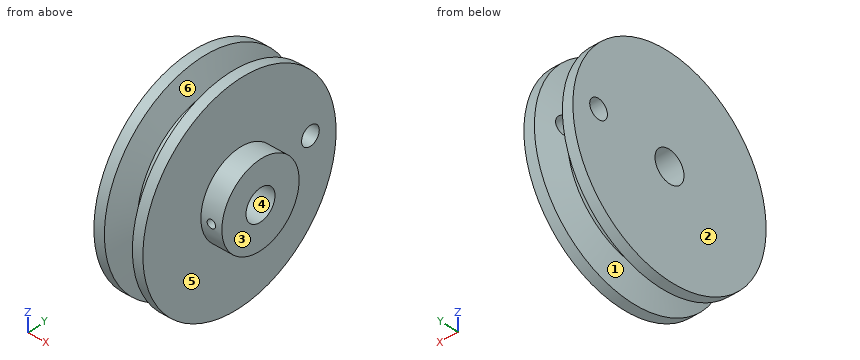
from build123d import *

# Parameters (mm, degrees)
F3_D     = 5.5
F3_DEPTH = 14
F3_TIP   = 1.6523667023
F6_D     = 2.4
F6_DEPTH = 13.4
F6_TIP   = 0.7210327428


with BuildPart() as f1:
    # F0 (on Front) → F1 (revolve)
    with BuildSketch(Plane.XZ):
        Polygon((-7, 30), (-7, 4.5), (13, 4.5), (13, 12), (7, 12), (7, 30), (4, 30), (1.9940651348, 21.9546346889), (-2.0053759773, 22), (-4, 30), align=None)
    revolve(axis=Axis((0, 0, 0), (1, 0, 0)))

    # F3
    with Locations(Plane(origin=(-7, 0, 0), x_dir=(0, -1, 0), z_dir=(-1, 0, 0))):
        with Locations((-22.0234822482, 3.0874926597)):
            Hole(F3_D / 2, depth=F3_DEPTH)
            with Locations((0, 0, -(F3_DEPTH + F3_TIP / 2))):  # 118° drill point
                Cone(0, F3_D / 2, F3_TIP, mode=Mode.SUBTRACT)

    # F6
    with Locations(Plane.XZ.offset(12)):
        with Locations((10, 0)):
            Hole(F6_D / 2, depth=F6_DEPTH)
            with Locations((0, 0, -(F6_DEPTH + F6_TIP / 2))):  # 118° drill point
                Cone(0, F6_D / 2, F6_TIP, mode=Mode.SUBTRACT)


solid = f1.part
Verification items for the finished model (mm, model axes). Face numbers are marked on the shaded views. A direction names the side the tool comes from. Coordinates: 2 decimals unless noted, no trailing zeros. Order: outer loops, then holes, each group sorted by start corner. A loop starts at its lowest first (then second) coordinate and runs counter-clockwise, first axis right, second up. Notation, with made-up numbers: (86.25, 77) -> (133.25, 77) arc R21 ccw to (133.25, 90) -> close; hole circle Ø5 at (-17.5, -9). An arc over 180 degrees is marked (long way). Put each result on its own line as item: value. Start each with the question number.
1. Mould release check, pull along X, two halves, no side actions. Record for the marked faces 1, 2 and 3: released by +X, released by -X, zero draft, split by the parting line, or undercut.
2. Access from +Z, -Z, +X, -X, +Y, -Y to the whole of each face (thin tool, end or side, straight path). Record for the marked faces 4, 5 and 6.
3. Cross-section at A-A, the plane x = -0.25. Record the boundary of the cut face in (y, z), then the cut area to 3 significant figures.
4. Material ranges on L1, parallel to Z at x = 8.75, y = 0; L2, parallel to X at y = -9, z = 0; L3, parallel to X at y = 15, z = 6.5, recorded low to high. Write a range as [from, to].
5. Cross-section at B-B, the plane x = 10. Record the boundary of the cut face in (y, z), then the cut area to 3 significant figures.
6. Go/stop test with flat-tipped pins: pin 1 Ø1 at (x, z) = (10.5, 11.5) entering from -Y; pin 2 Ø3 at (x, z) = (10, 0) entering from -Y; pin 3 Ø3 at (y, z) = (2, 20) entering from +X; pin 4 Ø3.5 at (y, z) = (22.02, 3.09) entering from +X. Record where each tip stops, or that it passes through.
Computed:
1. face 1: undercut
1. face 2: released by -X
1. face 3: released by +X
2. face 4: +X, -X
2. face 5: +X
2. face 6: none
3. outline: (21.22, 5.72) arc R21.98 ccw (long way) to (21.98, 0.34) arc R2.75 cw to start; hole circle Ø9 at (0, 0)
3. area: 1,440 mm2
4. L1: [-12, -4.5], [4.5, 12]
4. L2: [-7, 8.8], [11.2, 13]
4. L3: [-7, 7]
5. outline: (-11.94, -1.2) arc R12 ccw (long way) to (-11.94, 1.2) -> (-4.34, 1.2) arc R4.5 cw (long way) to (-4.34, -1.2) -> close
5. area: 371 mm2
6. pin 1: y = -4.8
6. pin 2: y = -12
6. pin 3: x = 7
6. pin 4: through
